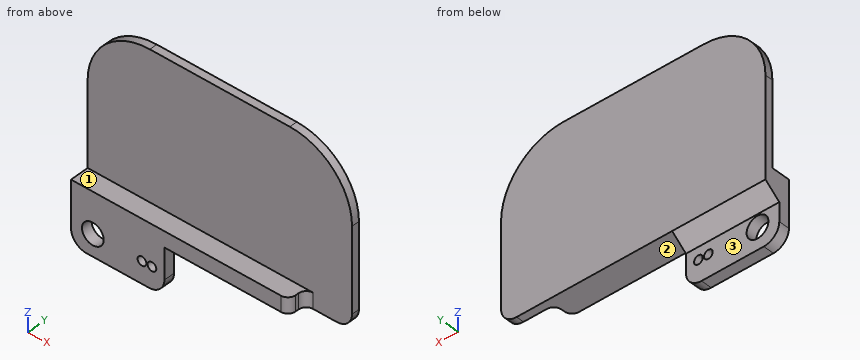
from build123d import *

# Parameters (mm, degrees)
SKETCH1_W           = 107.95
SKETCH1_H           = 85.09
SKETCH1_R           = 4.445
BOSS_EXTRUDE1_DEPTH = 3.175
SKETCH2_W           = 107.95
SKETCH2_H           = 25.4
SKETCH2_R           = 4.445
BOSS_EXTRUDE2_DEPTH = 7.62
SKETCH3_W           = 69.85
SKETCH3_H           = 19.05
CUT_EXTRUDE1_DEPTH  = 11.795
SKETCH4_W           = 38.1
SKETCH4_H           = 19.05
CUT_EXTRUDE2_DEPTH  = 6.35
SKETCH5_R           = 1.778
CUT_EXTRUDE3_DEPTH  = 5.445
SKETCH6_W           = 19.05
SKETCH6_H           = 7.62
CUT_EXTRUDE4_DEPTH  = 26.4
BOSS_EXTRUDE3_DEPTH = 38.1
FILLET1_R           = 25.4
FILLET2_R           = 6.35
FILLET3_R           = 3.175


with BuildPart() as part:
    # Sketch1 → Boss-Extrude1 (new body)
    with BuildSketch(Plane(origin=(0, 0, 0), x_dir=(1, 0, 0), z_dir=(0, 1, 0))):
        with Locations((53.975, 42.545)):
            Rectangle(SKETCH1_W, SKETCH1_H)
        with Locations((8.89, 76.2)):
            Circle(SKETCH1_R, mode=Mode.SUBTRACT)
    extrude(amount=BOSS_EXTRUDE1_DEPTH)

    # Sketch2 → Boss-Extrude2 (add)
    with BuildSketch(Plane.XZ):
        with Locations((53.975, -72.39)):
            Rectangle(SKETCH2_W, SKETCH2_H)
        with Locations((8.89, -76.2)):
            Circle(SKETCH2_R, mode=Mode.SUBTRACT)
    extrude(amount=BOSS_EXTRUDE2_DEPTH)

    # Sketch3 → Cut-Extrude1 (cut, through all)
    with BuildSketch(Plane.XZ.offset(7.62)):
        with Locations((73.025, -75.565)):
            Rectangle(SKETCH3_W, SKETCH3_H)
    extrude(amount=-CUT_EXTRUDE1_DEPTH, mode=Mode.SUBTRACT)

    # Sketch4 → Cut-Extrude2 (cut)
    with BuildSketch(Plane(origin=(0, 3.175, 0), x_dir=(1, 0, 0), z_dir=(0, 1, 0))):
        with Locations((19.05, 75.565)):
            Rectangle(SKETCH4_W, SKETCH4_H)
    extrude(amount=-CUT_EXTRUDE2_DEPTH, mode=Mode.SUBTRACT)

    # Sketch5 → Cut-Extrude3 (cut, through all)
    with BuildSketch(Plane(origin=(0, -3.175, 0), x_dir=(1, 0, 0), z_dir=(0, 1, 0))):
        with Locations((28.956, 76.2)):
            Circle(SKETCH5_R)
        with Locations((33.02, 76.2)):
            Circle(SKETCH5_R)
    extrude(amount=-CUT_EXTRUDE3_DEPTH, mode=Mode.SUBTRACT)

    # Sketch6 → Cut-Extrude4 (cut, through all)
    with BuildSketch(Plane.XY.offset(-59.69)):
        with Locations((98.425, -3.81)):
            Rectangle(SKETCH6_W, SKETCH6_H)
    extrude(amount=-CUT_EXTRUDE4_DEPTH, mode=Mode.SUBTRACT)

    # Sketch7 → Boss-Extrude3 (add)
    with BuildSketch(Plane.ZY):
        Polygon((-66.04, 3.175), (-71.12, -3.175), (-66.04, -3.175), align=None)
    extrude(amount=-BOSS_EXTRUDE3_DEPTH)

    # Fillet1
    fillet1_edges = [part.edges().sort_by_distance(p)[0] for p in [
        (107.95, 1.5875, 0),
        (0, 1.5875, 0),
    ]]
    fillet(fillet1_edges, radius=FILLET1_R)

    # Fillet2
    fillet2_edges = [part.edges().sort_by_distance(p)[0] for p in [
        (107.95, 1.5875, -66.04),
        (38.1, -5.3975, -85.09),
        (0, -5.3975, -85.09),
    ]]
    fillet(fillet2_edges, radius=FILLET2_R)

    # Fillet3
    fillet3_edges = [part.edges().sort_by_distance(p)[0] for p in [
        (88.9, -7.62, -62.865),
        (88.9, 0, -62.865),
    ]]
    fillet(fillet3_edges, radius=FILLET3_R)


solid = part.part
Geometry check sheet. Reference: the model listing, model coordinates, mm. Face numbers are marked on the shaded views. A direction names the side the tool comes from. Coordinates: 2 decimals unless noted, no trailing zeros. Order: outer loops, then holes, each group sorted by start corner. A loop starts at its lowest first (then second) coordinate and runs counter-clockwise, first axis right, second up. Notation, with made-up numbers: (38.25, 61.5) - (61.25, 61.5) arc R13 ccw to (61.25, 78.5) - close; hole circle Ø9 at (35.25, -7). An arc over 180 degrees is marked (long way). Answer in a Markdown table with one row per item. Add a question column.
1) Cross-section at C-C, the plane x = 67. Record the cut outline in (y, z) (3 decimals).
2) Set-up check for the marked faces 1, 2 and 3: record each of +Z, -Z, +X, -X, +Y, -Y from which the full face is reachable in a straight line by a thin tool's end or side.
3) Cross-section at D-D, the plane z = -62.5. Record the cut outline in (x, y) (3 decimals).
4) Gauge pin test, flat ends, axial feed: P1, Ø4.5, axis at x = 33.02, z = -76.2, coming from the -Y side; P2, Ø1, axis at x = 75.5, z = -41, coming from the -Y side; P3, Ø4, axis at x = 11.5, z = -81, coming from the +Y side (3 decimals); P4, Ø6, axis at x = 32, y = -3.5, coming from the +Z side. Record the tip position at first contact, or that the pin passes through.
5) Cross-section at A-A, the plane z = -76.2. Record the cut outline in (x, y) (3 decimals), then the cut area to 3 significant figures.
6) Cross-section at B-B, the plane x = 33.02. Record the cut outline in (y, z) (3 decimals).
7) Material ranges on line 1 along X through (y, z) = (-4.7, -76.2) (3 decimals); line 2 along Z through (x, y) = (8.89, -5.85) (3 decimals); line 3 along Z through (x, y) = (59, -6.25), recorded low to high. Write a range as [from, to].
Check result:
| question | item | result |
|---|---|---|
| 1 | outline | (-7.62, -66.04) - (3.175, -66.04) - (3.175, 0) - (0, 0) - (0, -59.69) - (-7.62, -59.69) - close |
| 2 | face 1 | +Z, +X, -X, -Y |
| 2 | face 2 | -Z, +X, +Y, -Y |
| 2 | face 3 | -Z, +X, -X, +Y |
| 3 | outline | (0, -7.62) - (85.725, -7.62) arc R3.175 ccw to (88.9, -4.445) - (88.9, -3.175) arc R3.175 cw to (92.075, 0) - (107.294, 0) - (107.294, 3.175) - (0, 3.175) - close |
| 4 | P1 | stops at y = -7.62 |
| 4 | P2 | stops at y = 0 |
| 4 | P3 | stops at y = -3.175 |
| 4 | P4 | stops at z = -59.69 |
| 5 | outline | (0, -7.62) - (4.445, -7.62) - (4.445, -3.175) - (0, -3.175) - close; (13.335, -7.62) - (27.178, -7.62) - (27.178, -3.175) - (13.335, -3.175) - close; (30.734, -7.62) - (31.242, -7.62) - (31.242, -3.175) - (30.734, -3.175) - close; (34.798, -7.62) - (38.1, -7.62) - (38.1, -3.175) - (34.798, -3.175) - close |
| 5 | area | 98.2 mm² |
| 6 | outline | (-7.62, -84.962) - (-3.175, -84.962) - (-3.175, -77.978) - (-7.62, -77.978) - close; (-7.62, -74.422) - (-3.175, -74.422) - (-3.175, -71.12) - (3.175, -66.04) - (3.175, 0) - (0, 0) - (0, -59.69) - (-7.62, -59.69) - close |
| 7 | line 1 | x = [0, 4.445], [13.335, 27.178], [30.734, 31.242], [34.798, 38.1] |
| 7 | line 2 | z = [-85.09, -80.645], [-71.755, -59.69] |
| 7 | line 3 | z = [-66.04, -59.69] |
